The model under review builds one solid part; all positions refer to its coordinate system, in mm. A direction names the side the tool comes from. Give positions to 0.01 mm unless a question says otherwise; leave off trailing zeros. Order: outer loops, then holes, each group sorted by start corner. A loop starts at its lowest first (then second) coordinate and runs counter-clockwise, first axis right, second up.
```python
from build123d import *

# Parameters (mm, degrees)
SKETCH2_W           = 43
SKETCH2_H           = 100
BOSS_EXTRUDE1_DEPTH = 54
SKETCH3_W           = 83
SKETCH3_H           = 100
BOSS_EXTRUDE2_DEPTH = 91
SKETCH4_W           = 16
SKETCH4_H           = 100
BOSS_EXTRUDE3_DEPTH = 66
SKETCH6_W           = 39
SKETCH6_H           = 100
BOSS_EXTRUDE4_DEPTH = 100
SKETCH5_W           = 6
SKETCH5_H           = 35
CUT_EXTRUDE1_DEPTH  = 200
SKETCH7_W           = 39
SKETCH7_H           = 100
BOSS_EXTRUDE5_DEPTH = 1


with BuildPart() as part:
    # Sketch2 → Boss-Extrude1 (new body)
    with BuildSketch(Plane.XY):
        Rectangle(SKETCH2_W, SKETCH2_H)
    extrude(amount=BOSS_EXTRUDE1_DEPTH)

    # Sketch3 → Boss-Extrude2 (add)
    with BuildSketch(Plane.XY):
        with Locations((63, 0)):
            Rectangle(SKETCH3_W, SKETCH3_H)
    extrude(amount=BOSS_EXTRUDE2_DEPTH)

    # Sketch4 → Boss-Extrude3 (add)
    with BuildSketch(Plane.XY):
        with Locations((112.5, 0)):
            Rectangle(SKETCH4_W, SKETCH4_H)
    extrude(amount=BOSS_EXTRUDE3_DEPTH)

    # Sketch6 → Boss-Extrude4 (add)
    with BuildSketch(Plane.XY):
        with Locations((140, 0)):
            Rectangle(SKETCH6_W, SKETCH6_H)
    extrude(amount=BOSS_EXTRUDE4_DEPTH)

    # Sketch5 → Cut-Extrude1 (cut)
    with BuildSketch(Plane(origin=(159.5, 0, 0), x_dir=(0, 0, -1), z_dir=(1, 0, 0))):
        with Locations((-3, -13.5)):
            Rectangle(SKETCH5_W, SKETCH5_H)
    extrude(amount=-CUT_EXTRUDE1_DEPTH, mode=Mode.SUBTRACT)

    # Sketch7 → Boss-Extrude5 (add)
    with BuildSketch(Plane.XZ.offset(50)):
        with Locations((140, 50)):
            Rectangle(SKETCH7_W, SKETCH7_H)
    extrude(amount=BOSS_EXTRUDE5_DEPTH)


solid = part.part
```
Item 1: Take a section at B-B (y = -27.5). Give the boundary of the cut face in (x, z).
Values found:
outline: (-21.5, 6) - (159.5, 6) - (159.5, 100) - (120.5, 100) - (120.5, 66) - (104.5, 66) - (104.5, 91) - (21.5, 91) - (21.5, 54) - (-21.5, 54) - close
Item 2: Take a section at C-C (x = 6). Give the boundary of the cut face in (y, z).
Values found:
outline: (-50, 0) - (-31, 0) - (-31, 6) - (4, 6) - (4, 0) - (50, 0) - (50, 54) - (-50, 54) - close
Item 3: For faces 4 (the flat face through (104.5, -1, 78)), 5 (the flat face through (70, 4, 3)), 6 (the flat face through (68, 27, 0)), 7 (the flat face through (21.5, -1, 72)), list the 3-axis set-ups (+Z, -Z, +X, -X, +Y, -Y) from which the entire face can be reached by the end or side of a thin tool; tool diameter is ignored.
Values found:
face 4: +Z, +Y, -Y
face 5: -Z, +X, -X
face 6: -Z, +X, -X, +Y, -Y
face 7: +Z, -X, +Y, -Y
Item 4: Take a section at A-A (z = 76.5). Give the boundary of the cut face in (x, y), and give its area (3 significant figures).
Values found:
outline: (21.5, -50) - (104.5, -50) - (104.5, 50) - (21.5, 50) - close; (120.5, -51) - (159.5, -51) - (159.5, 50) - (120.5, 50) - close
area: 12,200 mm2
Item 5: Clearance check with flat-ended pins moving along their axes: pin 1 Ø10 at (x, z) = (79, 28) entering from -Y; pin 2 Ø8 at (x, y) = (73, 7.5) entering from +Z; pin 3 Ø1 at (x, y) = (-3, -30.5) entering from +Z; pin 4 Ø3 at (x, y) = (47, 21.5) entering from -Z. State where each tip first meets the part, or that it passes through.
Values found:
pin 1: stops at y = -50
pin 2: stops at z = 91
pin 3: stops at z = 54
pin 4: stops at z = 0
Item 6: Draft analysis for pull direction Y (two halves, no side actions). For faces 1 (the flat face through (70, -14, 6)), 2 (the flat face through (140, 0, 100)), 3 (the flat face through (49, -50, 35)), state which applies: released by +Y, released by -Y, zero draft, split by the parting line, or undercut.
Values found:
face 1: undercut
face 2: zero draft
face 3: released by -Y
Item 7: Take a section at D-D (y = 20). Give the boundary of the cut face in (x, z).
Values found:
outline: (-21.5, 0) - (159.5, 0) - (159.5, 100) - (120.5, 100) - (120.5, 66) - (104.5, 66) - (104.5, 91) - (21.5, 91) - (21.5, 54) - (-21.5, 54) - close
Item 8: For line 1 (X direction, y = 11, z = 72); line 2 (Z direction, x = 57, y = -42.5); line 3 (Y direction, x = 111, z = 55), list the stretches that pass through material, from the lowest coordinate up.
Values found:
line 1: x = 21.5 to 104.5, 120.5 to 159.5
line 2: z = 0 to 91
line 3: y = -50 to 50
